from build123d import *

# Parameters (mm, degrees)
BOSS_EXTRUDE1_DEPTH     = 7.5
BOSS_EXTRUDE1_2_DEPTH   = 7.5
BOSS_EXTRUDE1_3_DEPTH   = 7.5
BOSS_EXTRUDE1_4_DEPTH   = 7.5
SKETCH1_3_W             = 25
SKETCH1_3_H             = 25
SKETCH1_3_R             = 5.05
BOSS_EXTRUDE2_DEPTH     = 15
BOSS_EXTRUDE5_DEPTH     = 7.5
BOSS_EXTRUDE8_DEPTH     = 15
SKETCH1_8_R             = 17.67766953
BOSS_EXTRUDE9_DEPTH     = 40
BOSS_EXTRUDE10_DEPTH    = 20
CUT_EXTRUDE1_DEPTH      = 94.808315196
CUT_EXTRUDE1_DEPTH_BACK = 94.808315196
SKETCH1_9_R             = 5.05


# Read off the part's stored shape, not the designer's step: Boss-Extrude5
with BuildPart() as part:
    # Sketch1 → Boss-Extrude1 (new body)
    with BuildSketch(Plane(origin=(0, 0, 0), x_dir=(1, 0, 0), z_dir=(0, 1, 0))):
        with BuildLine():
            Line((-60, 12.5), (-60, -12.5))
            Line((-60, -12.5), (-12.5, -12.5))
            ThreePointArc((-12.5, -12.5), (-17.67766953, 0), (-12.5, 12.5))
            Line((-12.5, 12.5), (-60, 12.5))
        make_face()
    extrude(amount=BOSS_EXTRUDE1_DEPTH)



with BuildPart() as body_2:
    # Sketch1 → Boss-Extrude1 2 (new body)
    with BuildSketch(Plane(origin=(0, 0, 0), x_dir=(1, 0, 0), z_dir=(0, 1, 0))):
        with BuildLine():
            ThreePointArc((12.5, -12.5), (0, -17.67766953), (-12.5, -12.5))
            Line((-12.5, -12.5), (-12.5, -60))
            Line((-12.5, -60), (12.5, -60))
            Line((12.5, -60), (12.5, -12.5))
        make_face()
    extrude(amount=BOSS_EXTRUDE1_2_DEPTH)


with BuildPart() as body_3:
    # Sketch1 → Boss-Extrude1 3 (new body)
    with BuildSketch(Plane(origin=(0, 0, 0), x_dir=(1, 0, 0), z_dir=(0, 1, 0))):
        with BuildLine():
            ThreePointArc((12.5, 12.5), (17.67766953, 0), (12.5, -12.5))
            Line((12.5, -12.5), (60, -12.5))
            Line((60, -12.5), (60, 12.5))
            Line((60, 12.5), (12.5, 12.5))
        make_face()
    extrude(amount=BOSS_EXTRUDE1_3_DEPTH)


with BuildPart() as body_4:
    # Sketch1 → Boss-Extrude1 4 (new body)
    with BuildSketch(Plane(origin=(0, 0, 0), x_dir=(1, 0, 0), z_dir=(0, 1, 0))):
        with BuildLine():
            Line((-12.5, 60), (-12.5, 12.5))
            ThreePointArc((-12.5, 12.5), (0, 17.67766953), (12.5, 12.5))
            Line((12.5, 12.5), (12.5, 60))
            Line((12.5, 60), (-12.5, 60))
        make_face()
    extrude(amount=BOSS_EXTRUDE1_4_DEPTH)


with BuildPart() as body_5:
    # Sketch1<3> → Boss-Extrude2 (new body)
    with BuildSketch(Plane(origin=(0, 0, 0), x_dir=(1, 0, 0), z_dir=(0, 1, 0))):
        Rectangle(SKETCH1_3_W, SKETCH1_3_H)
        with Locations(Location((0, 0, 0), (0, 0, 270))):
            Circle(SKETCH1_3_R, mode=Mode.SUBTRACT)
    extrude(amount=BOSS_EXTRUDE2_DEPTH)


with BuildPart() as body_6:
    # Boss-Extrude5 outline → Boss-Extrude5 (new body)
    with BuildSketch(Plane(origin=(0, 0, 0), x_dir=(1, 0, 0), z_dir=(0, 1, 0))):
        with BuildLine():
            Line((-12.5, 60), (-12.5, 12.5))
            ThreePointArc((-12.5, 12.5), (0, 17.67766953), (12.5, 12.5))
            Line((12.5, 12.5), (12.5, 60))
            Line((12.5, 60), (-12.5, 60))
        make_face()
    extrude(amount=BOSS_EXTRUDE5_DEPTH)


with BuildPart() as part_1:
    add(part.part)

    add(body_2.part)  # Boss-Extrude8 merges body 2

    add(body_3.part)  # Boss-Extrude8 merges body 3

    add(body_4.part)  # Boss-Extrude8 merges body 4

    add(body_5.part)  # Boss-Extrude8 merges body 5

    add(body_6.part)  # Boss-Extrude8 merges body 6
    # Sketch1<7> → Boss-Extrude8 (add)
    with BuildSketch(Plane(origin=(0, 0, 0), x_dir=(1, 0, 0), z_dir=(0, 1, 0))):
        with BuildLine():
            ThreePointArc((-12.5, 12.5), (-17.67766953, 0), (-12.5, -12.5))
            Line((-12.5, -12.5), (-12.5, 12.5))
        make_face()
        with BuildLine():
            Line((12.5, -12.5), (-12.5, -12.5))
            ThreePointArc((-12.5, -12.5), (0, -17.67766953), (12.5, -12.5))
        make_face()
        with BuildLine():
            Line((12.5, 12.5), (12.5, -12.5))
            ThreePointArc((12.5, -12.5), (16.332037061, -6.764951252), (17.67766953, 0))
            ThreePointArc((17.67766953, 0), (16.332037061, 6.764951252), (12.5, 12.5))
        make_face()
        with BuildLine():
            ThreePointArc((12.5, 12.5), (0, 17.67766953), (-12.5, 12.5))
            Line((-12.5, 12.5), (12.5, 12.5))
        make_face()
    extrude(amount=BOSS_EXTRUDE8_DEPTH)

    # Sketch1<8> → Boss-Extrude9 (add)
    with BuildSketch(Plane(origin=(0, 0, 0), x_dir=(1, 0, 0), z_dir=(0, 1, 0))):
        with Locations(Location((0, 0, 0), (0, 0, 45))):
            Circle(SKETCH1_8_R)
    extrude(amount=BOSS_EXTRUDE9_DEPTH)

    # Sketch5 → Boss-Extrude10 (add)
    with BuildSketch(Plane(origin=(0, 7.5, 0), x_dir=(1, 0, 0), z_dir=(0, 1, 0))):
        with BuildLine():
            Line((-60, 7.5), (-16.007810594, 7.5))
            ThreePointArc((-16.007810594, 7.5), (-14.471482861, 10.152644177), (-12.5, 12.5))
            Line((-12.5, 12.5), (-60, 12.5))
            Line((-60, 12.5), (-60, 7.5))
        make_face()
        with BuildLine():
            Line((-12.5, 60), (-12.5, 12.5))
            ThreePointArc((-12.5, 12.5), (-10.152644177, 14.471482861), (-7.5, 16.007810594))
            Line((-7.5, 16.007810594), (-7.5, 60))
            Line((-7.5, 60), (-12.5, 60))
        make_face()
        with BuildLine():
            Line((7.5, 60), (7.5, 16.007810594))
            ThreePointArc((7.5, 16.007810594), (10.152644177, 14.471482861), (12.5, 12.5))
            Line((12.5, 12.5), (12.5, 60))
            Line((12.5, 60), (7.5, 60))
        make_face()
        with BuildLine():
            ThreePointArc((12.5, 12.5), (14.471482861, 10.152644177), (16.007810594, 7.5))
            Line((16.007810594, 7.5), (60, 7.5))
            Line((60, 7.5), (60, 12.5))
            Line((60, 12.5), (12.5, 12.5))
        make_face()
        with BuildLine():
            ThreePointArc((16.007810594, -7.5), (14.471482861, -10.152644177), (12.5, -12.5))
            Line((12.5, -12.5), (60, -12.5))
            Line((60, -12.5), (60, -7.5))
            Line((60, -7.5), (16.007810594, -7.5))
        make_face()
        with BuildLine():
            ThreePointArc((12.5, -12.5), (10.152644177, -14.471482861), (7.5, -16.007810594))
            Line((7.5, -16.007810594), (7.5, -60))
            Line((7.5, -60), (12.5, -60))
            Line((12.5, -60), (12.5, -12.5))
        make_face()
        with BuildLine():
            ThreePointArc((-7.5, -16.007810594), (-10.152644177, -14.471482861), (-12.5, -12.5))
            Line((-12.5, -12.5), (-12.5, -60))
            Line((-12.5, -60), (-7.5, -60))
            Line((-7.5, -60), (-7.5, -16.007810594))
        make_face()
        with BuildLine():
            Line((-60, -12.5), (-12.5, -12.5))
            ThreePointArc((-12.5, -12.5), (-14.471482861, -10.152644177), (-16.007810594, -7.5))
            Line((-16.007810594, -7.5), (-60, -7.5))
            Line((-60, -7.5), (-60, -12.5))
        make_face()
    extrude(amount=BOSS_EXTRUDE10_DEPTH)

    # Sketch1<9> → Cut-Extrude1 (cut, two sides: drawn at the far end of the back side and taken through both)
    with BuildSketch(Plane(origin=(0, 0, 0), x_dir=(1, 0, 0), z_dir=(0, 1, 0)).offset(-CUT_EXTRUDE1_DEPTH_BACK)):
        with Locations(Location((0, 0, 0), (0, 0, 270))):
            Circle(SKETCH1_9_R)
    extrude(amount=CUT_EXTRUDE1_DEPTH + CUT_EXTRUDE1_DEPTH_BACK, mode=Mode.SUBTRACT)


solid = part_1.part
Check sheet for the modelled part. Datum: model origin and axes. Units: mm. A direction names the side the tool comes from. Give positions to 0.01 mm unless a question says otherwise; leave off trailing zeros. Write each loop counter-clockwise with the first axis right and the second up, starting at its lowest first coordinate (ties: lowest second). Pieces come first, ordered by that corner, then holes. Notation, with made-up numbers: M 34,7 L 40,7 A24 ccw 40,19 Z; hole C 51,27 d11. An arc over 180 degrees is marked long. Use one line per item in the form item = value.
(1) Section check A-A on z = 0. Record the boundary of the cut face in (x, y).
Answer block:
outline = M -60,0 L -5.05,0 L -5.05,40 L -17.68,40 L -17.68,7.5 L -60,7.5 Z; M 5.05,0 L 60,0 L 60,7.5 L 17.68,7.5 L 17.68,40 L 5.05,40 Z
(2) Depth check by flat-ended pin: P1, Ø22, axis at y = 8.5, z = -25.5, coming from the -X side; P2, Ø2.5, axis at x = -11, z = 24.5, coming from the +Y side; P3, Ø3, axis at x = 42, y = 20, coming from the +Z side; P4, Ø12, axis at x = 5, z = -34.5, coming from the -Y side. Enter the tip coordinate at first touch or a pass-through.
Answer block:
P1 = -12.5
P2 = 27.5
P3 = 12.5
P4 = 0
(3) Section check D-D on z = 33.5. Record the boundary of the cut face in (x, y).
Answer block:
outline = M -12.5,0 L 12.5,0 L 12.5,27.5 L 7.5,27.5 L 7.5,7.5 L -7.5,7.5 L -7.5,27.5 L -12.5,27.5 Z
(4) Section check B-B on x = 0. Record the boundary of the cut face in (y, z).
Answer block:
outline = M 0,-60 L 7.5,-60 L 7.5,-17.68 L 40,-17.68 L 40,-5.05 L 0,-5.05 Z; M 0,5.05 L 40,5.05 L 40,17.68 L 7.5,17.68 L 7.5,60 L 0,60 Z
(5) Material ranges on line 1 along X through (y, z) = (14.5, 0); line 2 along X through (y, z) = (21.5, 46), recorded low to high.
Answer block:
line_1 = -17.68 to -5.05, 5.05 to 17.68
line_2 = -12.5 to -7.5, 7.5 to 12.5
(6) Draft check along X on faces 1 (the flat face through (60, 7, 0)), 2 (the flat face through (0, 7.5, -38)), 3 (the flat face through (36, 27.5, -10)). Enter one of: pulls with the +X half, pulls with the -X half, needs draft (parallel to the pull), parting line crosses it, or undercut.
Answer block:
face_1 = pulls with the +X half
face_2 = undercut
face_3 = needs draft
(7) Tool access check on faces 4 (the flat face through (-7.5, 17, 38)), 5 (the flat face through (-12.5, 14, 36)), 6 (the flat face through (37, 14, -12.5)). Record the directions out of +Z, -Z, +X, -X, +Y, -Y that give a thin tool (end or side, any length) a straight path to the whole face; none if there is none.
Answer block:
face_4 = +Z, +Y
face_5 = +Z, -X, +Y, -Y
face_6 = -Z, +X, +Y, -Y
